```python
from build123d import *

# Parameters (mm, degrees)
SKETCH_1_W          = 23
SKETCH_1_H          = 11.5
EXTRUDE_1_DEPTH     = 15
EXTRUDE_START       = 15
SKETCH_2_W          = 32
SKETCH_2_H          = 11.5
EXTRUDE_2_DEPTH     = 1.5
SKETCH_3_W          = 23
SKETCH_3_H          = 11.5
EXTRUDE_3_DEPTH     = 19.65
SKETCH_4_R          = 1
CUT_EXTRUDE_1_DEPTH = 19.65
SKETCH_5_R          = 5.75
EXTRUDE_4_DEPTH     = 24
EXTRUDE_5_DEPTH     = 24
EXTRUDE_START_2     = 24
SKETCH_7_R          = 1.75
EXTRUDE_6_DEPTH     = 2


with BuildPart() as part:
    # 草图1 → 凸台-拉伸1 (new body)
    with BuildSketch(Plane(origin=(0, 0, 0), x_dir=(1, 0, 0), z_dir=(0, 1, 0))):
        Rectangle(SKETCH_1_W, SKETCH_1_H)
    extrude(amount=EXTRUDE_1_DEPTH)

    # 草图2 → 凸台-拉伸2 (add)
    with BuildSketch(Plane(origin=(0, 0, 0), x_dir=(1, 0, 0), z_dir=(0, 1, 0)).offset(EXTRUDE_START)):
        Rectangle(SKETCH_2_W, SKETCH_2_H)
    extrude(amount=EXTRUDE_2_DEPTH)

    # 草图3 → 凸台-拉伸3 (add)
    with BuildSketch(Plane(origin=(0, 0, 0), x_dir=(1, 0, 0), z_dir=(0, 1, 0))):
        Rectangle(SKETCH_3_W, SKETCH_3_H)
    extrude(amount=EXTRUDE_3_DEPTH)

    # 草图4 → 切除-拉伸1 (cut)
    with BuildSketch(Plane(origin=(0, 0, 0), x_dir=(1, 0, 0), z_dir=(0, 1, 0))):
        with Locations(Location((-13.8, 0, 0), (0, 0, 90))):
            Circle(SKETCH_4_R)
        with Locations(Location((13.8, 0, 0), (0, 0, 90))):
            Circle(SKETCH_4_R)
    extrude(amount=CUT_EXTRUDE_1_DEPTH, mode=Mode.SUBTRACT)

    # 草图5 → 凸台-拉伸4 (add)
    with BuildSketch(Plane(origin=(0, 0, 0), x_dir=(1, 0, 0), z_dir=(0, 1, 0))):
        with Locations(Location((-5.75, 0, 0), (0, 0, 270))):
            Circle(SKETCH_5_R)
    extrude(amount=EXTRUDE_4_DEPTH)

    # 草图6 → 凸台-拉伸5 (add)
    with BuildSketch(Plane(origin=(0, 0, 0), x_dir=(1, 0, 0), z_dir=(0, 1, 0))):
        with BuildLine():
            Line((-1.565217391, 3.943360815), (1.189071712, 2.754289103))
            ThreePointArc((1.189071712, 2.754289103), (3, 0), (1.189071712, -2.754289103))
            Line((1.189071712, -2.754289103), (-1.565217391, -3.943360815))
            ThreePointArc((-1.565217391, -3.943360815), (-11.5, 0), (-1.565217391, 3.943360815))
        make_face()
    extrude(amount=EXTRUDE_5_DEPTH)

    # 草图7 → 凸台-拉伸6 (add)
    with BuildSketch(Plane(origin=(0, 0, 0), x_dir=(1, 0, 0), z_dir=(0, 1, 0)).offset(EXTRUDE_START_2)):
        with Locations(Location((-5.75, 0, 0), (0, 0, 270))):
            Circle(SKETCH_7_R)
    extrude(amount=EXTRUDE_6_DEPTH)


solid = part.part
```
Part model, mm, in its own coordinate system. A direction names the side the tool comes from. Round coordinates to 2 decimals unless told otherwise and drop trailing zeros. Order: outer loops, then holes, each group sorted by start corner. A loop starts at its lowest first (then second) coordinate and runs counter-clockwise, first axis right, second up. Notation, with made-up numbers: M 30.25,77 L 40.25,77 A15 cw 40.25,95 Z; hole C 52.5,37.25 d2. An arc over 180 degrees is marked long. Answer in a Markdown table with one row per item. Add a question column.
Q1. Cut at A-A on x = 13.8. Give the cut face in (y, z), and give its area (4 significant figures).
Q2. Pin check, flat tips, straight feed: pin 1 (4.5 mm diameter, centred on x = -9, z = 3.5, fed in from +Y); pin 2 (3.5 mm diameter, centred on x = 13.5, z = -1, fed in from -Y); pin 3 (0.9 mm diameter, centred on y = 18.5, z = -1.5, fed in from +X). Stop position of each tip, or through.
Q3. Cut at C-C on y = 14. Give the cut face in (x, z).
Q4. Cut at B-B on x = -1. Give the cut face in (y, z).
Q5. Cut at D-D on z = -3.5. Give the cut face in (x, y), and give its area (3 significant figures).
Q6. 3-axis set-ups, long thin cutter, end or side, ignore diameter. For faces 1 (the face through (-11.5, 18, 0)), 2 (the face through (-13.8, 15, -1.4)), 3 (the face through (-0.21, 21.79, -3.36)): which of +Z, -Z, +X, -X, +Y, -Y reach the whole face in a straight line?
Q7. Wall check: L1, parallel to X at y = 15.8, z = 0; L2, parallel to Y at x = -7, z = -2.5; L3, parallel to X at y = 18, z = 2. Give the ranges that are in metal, low to high. Write a range as from..to.
Established:
| question | item | result |
|---|---|---|
| 1 | outline | M 15,-5.75 L 16.5,-5.75 L 16.5,-1 L 15,-1 Z; M 15,1 L 16.5,1 L 16.5,5.75 L 15,5.75 Z |
| 1 | area | 14.25 mm2 |
| 2 | pin 1 | stops at y = 24 |
| 2 | pin 2 | stops at y = 15 |
| 2 | pin 3 | stops at x = 11.5 |
| 3 | outline | M -11.5,-5.75 L 11.5,-5.75 L 11.5,5.75 L -11.5,5.75 Z |
| 4 | outline | M 0,-5.75 L 19.65,-5.75 L 19.65,-3.7 L 24,-3.7 L 24,3.7 L 19.65,3.7 L 19.65,5.75 L 0,5.75 Z |
| 5 | outline | M -16,15 L -11.5,15 L -11.5,0 L 11.5,0 L 11.5,15 L 16,15 L 16,16.5 L 11.5,16.5 L 11.5,19.65 L -0.54,19.65 L -0.54,24 L -10.31,24 L -10.31,19.65 L -11.5,19.65 L -11.5,16.5 L -16,16.5 Z |
| 5 | area | 508 mm2 |
| 6 | face 1 | +Z, -Z, -X, +Y |
| 6 | face 2 | +Z, -Z, -X, -Y |
| 6 | face 3 | -Z, +X, +Y |
| 7 | L1 | x = -16..-14.8, -12.8..12.8, 14.8..16 |
| 7 | L2 | y = 0..24 |
| 7 | L3 | x = -11.5..11.5 |
